```python
from build123d import *

# Parameters (mm, degrees)
SKETCH1_W           = 50
SKETCH1_H           = 54.105
BOSS_EXTRUDE1_DEPTH = 12
SKETCH2_R           = 3.15
CUT_EXTRUDE1_DEPTH  = 51
FILLET1_R           = 8
SKETCH3_R           = 12
SKETCH3_R_2         = 1.7
CUT_EXTRUDE2_DEPTH  = 13
CUT_EXTRUDE4_DEPTH  = 8


with BuildPart() as part:
    # Sketch1 → Boss-Extrude1 (new body)
    with BuildSketch(Plane.XY):
        with Locations((25, 27.0525)):
            Rectangle(SKETCH1_W, SKETCH1_H)
    extrude(amount=BOSS_EXTRUDE1_DEPTH)

    # Sketch2 → Cut-Extrude1 (cut, through all)
    with BuildSketch(Plane(origin=(0, 0, 0), x_dir=(0, 0, -1), z_dir=(1, 0, 0))):
        with Locations((-6, 46.105)):
            Circle(SKETCH2_R)
        with Locations((-6, 8)):
            Circle(SKETCH2_R)
    extrude(amount=CUT_EXTRUDE1_DEPTH, mode=Mode.SUBTRACT)

    # Fillet1
    fillet1_edges = [part.edges().sort_by_distance(p)[0] for p in [
        (25, 54.105, 0),
        (25, 0, 0),
    ]]
    fillet(fillet1_edges, radius=FILLET1_R)

    # Sketch3 → Cut-Extrude2 (cut, through all)
    with BuildSketch(Plane(origin=(0, 0, 0), x_dir=(-1, 0, 0), z_dir=(0, 0, -1))):
        with Locations((-32, 27.0525)):
            Circle(SKETCH3_R)
        with Locations((-19, 40.0525)):
            Circle(SKETCH3_R_2)
        with Locations((-19, 14.0525)):
            Circle(SKETCH3_R_2)
        with Locations((-45, 14.0525)):
            Circle(SKETCH3_R_2)
        with Locations((-45, 40.0525)):
            Circle(SKETCH3_R_2)
        with BuildLine():
            Line((-8.5, 0), (-8.5, 24.282572203))
            ThreePointArc((-8.5, 24.282572203), (-10.15, 27.0525), (-8.5, 29.822427797))
            Line((-8.5, 29.822427797), (-8.5, 33.0525))
            ThreePointArc((-8.5, 33.0525), (-7, 34.5525), (-5.5, 33.0525))
            Line((-5.5, 33.0525), (-5.5, 29.822427797))
            ThreePointArc((-5.5, 29.822427797), (-3.85, 27.0525), (-5.5, 24.282572203))
            Line((-5.5, 24.282572203), (-5.5, 0))
            Line((-5.5, 0), (-8.5, 0))
        make_face()
    extrude(amount=-CUT_EXTRUDE2_DEPTH, mode=Mode.SUBTRACT)

    # Sketch5 → Cut-Extrude4 (cut)
    with BuildSketch(Plane(origin=(0, 0, 0), x_dir=(-1, 0, 0), z_dir=(0, 0, -1))):
        with BuildLine():
            Line((-19, 17.6525), (-14, 17.6525))
            Line((-14, 17.6525), (-14, 36.4525))
            Line((-14, 36.4525), (-19, 36.4525))
            ThreePointArc((-19, 36.4525), (-21.510876341, 37.472674425), (-22.598679445, 39.955))
            Line((-22.598679445, 39.955), (-22.598679445, 41.7525))
            Line((-22.598679445, 41.7525), (-41.401320555, 41.7525))
            Line((-41.401320555, 41.7525), (-41.401320555, 39.955))
            ThreePointArc((-41.401320555, 39.955), (-42.489123659, 37.472674425), (-45, 36.4525))
            Line((-45, 36.4525), (-50, 36.4525))
            Line((-50, 36.4525), (-50, 17.6525))
            Line((-50, 17.6525), (-45, 17.6525))
            ThreePointArc((-45, 17.6525), (-42.489123659, 16.632325575), (-41.401320555, 14.15))
            Line((-41.401320555, 14.15), (-41.401320555, 12.3525))
            Line((-41.401320555, 12.3525), (-22.598679445, 12.3525))
            Line((-22.598679445, 12.3525), (-22.598679445, 14.15))
            ThreePointArc((-22.598679445, 14.15), (-21.510876341, 16.632325575), (-19, 17.6525))
        make_face()
    extrude(amount=-CUT_EXTRUDE4_DEPTH, mode=Mode.SUBTRACT)


solid = part.part
```
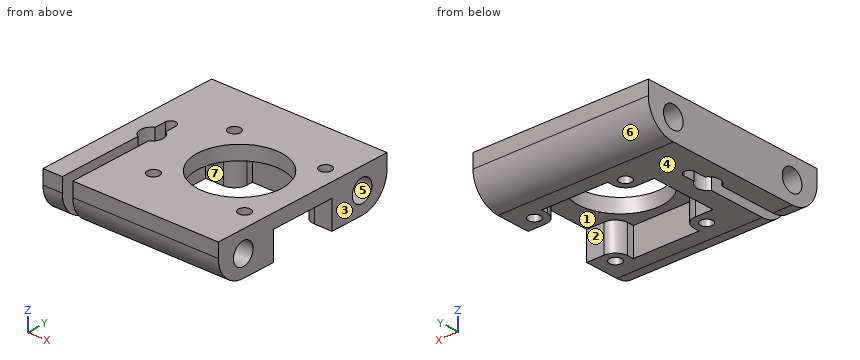
Source: CAD feature listing. Evaluate the final solid. Frame: model axes, mm. Face numbers are marked on the shaded views. A direction names the side the tool comes from. Give positions to 0.01 mm unless a question says otherwise; leave off trailing zeros. Write each loop counter-clockwise with the first axis right and the second up, starting at its lowest first coordinate (ties: lowest second). Pieces come first, ordered by that corner, then holes.
1. Section query B-B (y = 28.5). Return the cut outline in (x, z), then the cut area to 3 significant figures.
2. First-contact query: pin 1 (2.5 mm diameter, centred on x = 19, y = 40.05, fed in from -Z); pin 2 (2 mm diameter, centred on x = 32, z = 3.5, fed in from -Y); pin 3 (2.5 mm diameter, centred on x = 47, z = 4.5, fed in from +Y); pin 4 (2.5 mm diameter, centred on y = 31.5, z = 6.5, fed in from +X). Flat tips, straight axial feed; report the tip coordinate or a pass-through.
3. Section query A-A (x = 32). Count the separate pieces of the cut face and the enclosed holes in it, then the cut area to 3 significant figures.
4. Material intervals for line 1 along Y through (x, z) = (43, 4); line 2 along Z through (x, y) = (20.5, 8); line 3 along X through (y, z) = (11.5, 11.25), sorted ascending.
5. Section query C-C (x = 11.5). Return the cut outline in (y, z) (3 decimals), then the cut area to 3 significant figures.
6. Access query for the marked faces 1, 2 and 3. Directions: +Z, -Z, +X, -X, +Y, -Y. A direction counts if a zero-diameter tool reaches every point of the face in a straight line with its end or side. Return the directions, or none.
7. Pull-direction query (Y, two-part tool) for the marked faces 4, 5, 6 and 7; classes: +Y half, -Y half, draft (parallel to the pull), parting line (faces both ways), or undercut.
Output values:
1. outline: (0, 0) - (4.2, 0) - (4.2, 12) - (0, 12) - close; (9.8, 0) - (14, 0) - (14, 8) - (20.09, 8) - (20.09, 12) - (9.8, 12) - close; (43.91, 8) - (50, 8) - (50, 12) - (43.91, 12) - close
1. area: 150 mm2
2. pin 1: passes through
2. pin 2: stops at y = 0.81
2. pin 3: stops at y = 53.78
2. pin 4: stops at x = 14
3. separate pieces: 2
3. enclosed holes: 2
3. area: 228 mm2
4. line 1: y = 1.07 to 5.57, 10.43 to 17.05, 37.06 to 43.67, 48.54 to 53.03
4. line 2: z = 0 to 2.85, 9.15 to 12
4. line 3: x = 0 to 5.5, 8.5 to 50
5. outline: (0, 8) arc R8 ccw to (8, 0) - (46.105, 0) arc R8 ccw to (54.105, 8) - (54.105, 12) - (0, 12) - close; hole circle Ø6.3 at (8, 6); hole circle Ø6.3 at (46.105, 6)
5. area: 559 mm2
6. face 1: -Z
6. face 2: -Z, +X
6. face 3: +Z, -Z, +X, +Y, -Y
7. face 4: draft
7. face 5: undercut
7. face 6: +Y half
7. face 7: undercut
